Build history of the part. All positions in model axes, mm. A direction names the side the tool comes from. Give positions to 0.01 mm unless a question says otherwise; leave off trailing zeros. Loops run counter-clockwise (first coordinate to the right, second up) from the corner with the lowest first, then second, coordinate; pieces in that order, holes last. Notation, with made-up numbers: (-19, -5.5) - (7, -5.5) arc R24 cw to (7, 26.5) - close; hole circle Ø11 at (50.25, 48). An arc over 180 degrees is marked (long way). Return JSON: item names as keys, results as strings. Group by question number.
1) Slice it at B-B (x = -132.5). List the corners of the cut face in (y, z), and give its area (3 significant figures).
2) Drop flat-ended pins along their axis: pin 1 (0.9 mm diameter, centred on x = -199, z = -195, fed in from +Y); pin 2 (5 mm diameter, centred on x = -5, z = -200, fed in from +Y); pin 3 (9 mm diameter, centred on x = -5, z = -113, fed in from +Y). Give the stop position or say it passes through.
3) Slice it at A-A (z = -147). List the corners of the cut face in (x, y).
4) Mould opens along Z. For faces 6 (the face through (-190, 12, -180)), 7 (the face through (-196, 32, -101)), 8 (the face through (-200, 59, -93)) say: released by +Z, released by -Z, zero draft, split by the parting line, or undercut.
5) Slice it at C-C (y = 41). List the corners of the cut face in (x, z).
6) 3-axis set-ups, long thin cutter, end or side, ignore diameter. For faces 1 (the face through (-188, 15, -90)), 2 (the face through (-191.607, 1.232, -202.733)), 3 (the face through (-186.14, 17.675, -9.86)), 4 (the face through (-101, 0, -100)), 5 (the face through (-201.5, 18.8, -199.8)): which of +Z, -Z, +X, -X, +Y, -Y reach the whole face in a straight line?
7) Drill centre lines: probe 1 along Z at (x, y) = (-5, 1.6); probe 2 along X at (y, z) = (2, -200); probe 3 along Y at (x, z) = (-203.25, -201). Where is each one in solid material? Low to high. Write a range as from..to.
Autodesk Inventor part; units mm, degrees
ref_plane "YZ Plane" through (0, 0, 0) normal (1, 0, 0) x (0, 1, 0)
ref_plane "XZ Plane" through (0, 0, 0) normal (0, 1, 0) x (-1, 0, 0)
ref_plane "XY Plane" through (0, 0, 0) normal (0, 0, 1) x (1, 0, 0)
sketch "スケッチ1" plane through (0, 0, 0) normal (0, 1, 0) x (-1, 0, 0)
  line L0 (0, 0) -> (204, 0)
  line L1 (204, 0) -> (204, -205)
  line L2 (204, -205) -> (0, -205)
  line L3 (0, -205) -> (0, 0)
  dimension "d0" = 204
  dimension "d1" = 205
extrude "押し出し1" add sketch "スケッチ1" along normal blind 5
sketch "スケッチ2" plane through (0, 5, 0) normal (0, 1, 0) x (1, 0, 0)
  line L0 (-204, 205) -> (-204, 0)
  line L1 (0, 205) -> (-204, 205)
  line L2 (-204, 0) -> (-196, 0)
  line L3 (-196, 0) -> (-196, 205)
  line L4 (-196, 205) -> (-204, 205)
  line L5 (-204, 205) -> (-204, 0)
  point P0 (0, 0)
  dimension "d4" = 8
extrude "押し出し2" add sketch "スケッチ2" along normal blind 56
sketch "スケッチ3" plane through (0, 61, 0) normal (0, 1, 0) x (1, 0, 0)
  line L0 (-204, 205) -> (-204, 0)
  line L1 (-196, 0) -> (-196, 205)
  line L2 (-204, 0) -> (-196, 0)
  line L3 (-196, 0) -> (-196, 183)
  line L4 (-196, 183) -> (-204, 183)
  line L5 (-204, 183) -> (-204, 0)
  line L6 (-196, 205) -> (-204, 205)
  point P0 (0, 0)
  point P1 (-200, 183)
  dimension "d7" = 22
extrude "押し出し3" cut sketch "スケッチ3" against normal blind 2 contours L4 L1 L2 L0
sketch "スケッチ4" plane through (0, 61, 0) normal (0, 1, 0) x (1, 0, 0)
  circle A0 centre (-198.5, 195) radius 1.5
  line L0 (-196, 205) -> (-204, 205)
  line L1 (-196, 183) -> (-196, 205)
  line L2 (-204, 205) -> (-204, 183)
  point P0 (0, 0)
  dimension "d10" = 3
  dimension "d11" = 10
  dimension "d13" = 5.5
extrude "押し出し4" cut sketch "スケッチ4" against normal blind 10
sketch "スケッチ5" plane through (-204, 0, -205) normal (-1, 0, 0) x (0, 0, 1)
  circle A0 centre (4, 53) radius 1.5
  circle A1 centre (4, 20) radius 1.5
  line L0 (0, 61) -> (22, 61)
  line L1 (0, 0) -> (0, 61)
  point P0 (205, 0)
  dimension "d16" = 3
  dimension "d17" = 3
  dimension "d18" = 8
  dimension "d19" = 33
  dimension "d24" = 4
extrude "押し出し5" cut sketch "スケッチ5" against normal blind 10
sketch "スケッチ6" plane through (-204, 0, -205) normal (-1, 0, 0) x (0, 0, 1)
  circle A0 centre (4, 53) radius 1.5
  circle A1 centre (4, 53) radius 2.8
  circle A2 centre (4, 20) radius 1.5
  circle A3 centre (4, 20) radius 2.8
  point P0 (205, 0)
  dimension "d22" = 5.6
  dimension "d23" = 5.6
extrude "押し出し6" cut sketch "スケッチ6" against normal blind 2.5
sketch "スケッチ7" plane through (0, 0, 0) normal (0, -1, 0) x (1, 0, 0)
  circle A0 centre (-191, -200) radius 1.5
  circle A1 centre (-101, -200) radius 1.5
  circle A2 centre (-5, -200) radius 1.5
  line L0 (-204, 0) -> (0, 0)
  line L1 (0, 0) -> (0, -205)
  circle A3 centre (-5, -141) radius 1.5
  circle A4 centre (-5, -113) radius 1.5
  line L2 (0, -205) -> (-204, -205)
  dimension "d27" = 3
  dimension "d28" = 3
  dimension "d29" = 3
  dimension "d31" = 5
  dimension "d32" = 96
  dimension "d33" = 90
  dimension "d34" = 3
  dimension "d36" = 3
  dimension "d37" = 5
  dimension "d38" = 59
  dimension "d39" = 28
extrude "押し出し7" cut sketch "スケッチ7" against normal through all
sketch "スケッチ8" plane through (0, 0, 0) normal (0, -1, 0) x (1, 0, 0)
  circle A0 centre (-5, -113) radius 1.5
  circle A1 centre (-5, -113) radius 2.8
  circle A2 centre (-5, -141) radius 1.5
  circle A3 centre (-5, -141) radius 2.8
  circle A4 centre (-5, -200) radius 1.5
  circle A5 centre (-5, -200) radius 2.8
  circle A6 centre (-101, -200) radius 1.5
  circle A7 centre (-101, -200) radius 2.8
  circle A8 centre (-191, -200) radius 1.5
  circle A9 centre (-191, -200) radius 2.8
  point P0 (0, 0)
  dimension "d42" = 5.6
  dimension "d43" = 5.6
  dimension "d44" = 5.6
  dimension "d45" = 5.6
  dimension "d46" = 5.6
extrude "押し出し8" cut sketch "スケッチ8" against normal blind 2.5
sketch "スケッチ9" plane through (0, 5, 0) normal (0, 1, 0) x (1, 0, 0)
  line L0 (0, 205) -> (-204, 205)
  line L1 (0, 0) -> (-5, 0)
  line L2 (-5, 0) -> (-5, 205)
  line L3 (-5, 205) -> (0, 205)
  line L4 (0, 205) -> (0, 0)
  line L5 (-196, 183) -> (-196, 205)
  line L6 (0, 205) -> (-196, 205)
  line L7 (-196, 205) -> (-196, 200)
  line L8 (-196, 200) -> (0, 200)
  line L9 (0, 200) -> (0, 205)
  circle A0 centre (-5, 141) radius 1.5
  circle A1 centre (-5, 141) radius 3.1
  circle A2 centre (-5, 113) radius 1.5
  circle A3 centre (-5, 113) radius 4.1
  circle A4 centre (-5, 200) radius 1.5
  circle A5 centre (-5, 200) radius 3.1
  line L10 (-196, 205) -> (-185.8, 205)
  line L11 (-185.8, 205) -> (-185.8, 196.8)
  line L12 (-185.8, 196.8) -> (-196, 196.8)
  line L13 (-196, 196.8) -> (-196, 205)
  circle A6 centre (-101, 200) radius 1.5
  circle A7 centre (-101, 200) radius 3.1
  point P0 (-5, 137.9)
  point P1 (-5, 117.1)
  point P2 (-5, 108.9)
  point P3 (-185.8, 200)
  point P4 (-8.1, 200)
  point P5 (-5, 196.9)
  point P6 (-5, 144.1)
  point P7 (-104.1, 200)
  point P8 (-97.9, 200)
  point P9 (-99.5, 200)
  point P10 (-102.5, 200)
  dimension "d49" = 5
  dimension "d50" = 5
  dimension "d51" = 6.2
  dimension "d52" = 8.2
  dimension "d53" = 6.2
  dimension "d54" = 10.2
  dimension "d55" = 8.2
  dimension "d58" = 6.2
extrude "押し出し9" cut sketch "スケッチ9" against normal blind 1 contours L4 L8 A5 L2 L0 | L2 A5 L8 A7 L11 L0 | L4 L1 L2 A3 A1 A5 L8 | L11 L8 L5 L0 | A5 L8 A4 L2 | L2 A4 L8 A5 | A5 L2 A4 L8 | L11 L12 L5 L8 | A4 L8 L2 | L2 L8 A4 | L8 A4 L2 A5 | A4 L2 L8 | A7 L8 A6 | L8 A6 A7 | L2 A4 L8 | A3 L2 A2 | L2 A2 A3 | A1 L2 A0 | L2 A0 A1 | A6 L8 | A2 L2 | L2 A2 | A0 L2 | L2 A0 picked at (-100.9397, 200.4964)
sketch "スケッチ10" plane through (0, 5, 0) normal (0, 1, 0) x (1, 0, 0)
  line L0 (-196, 0) -> (-176, 0)
  line L1 (-176, 0) -> (-176, 20)
  line L2 (-176, 20) -> (-196, 20)
  line L3 (-196, 20) -> (-196, 0)
  line L4 (-196, 196.8) -> (-196, 0)
  line L5 (-196, 90) -> (-176, 90)
  line L6 (-176, 90) -> (-176, 100)
  line L7 (-176, 100) -> (-196, 100)
  line L8 (-196, 100) -> (-196, 90)
  line L9 (-196, 170) -> (-176, 170)
  line L10 (-176, 170) -> (-176, 180)
  line L11 (-176, 180) -> (-196, 180)
  line L12 (-196, 180) -> (-196, 170)
  point P0 (0, 0)
  dimension "d59" = 20
  dimension "d60" = 20
  dimension "d61" = 20
  dimension "d62" = 10
  dimension "d63" = 70
  dimension "d64" = 20
  dimension "d65" = 10
  dimension "d66" = 70
extrude "押し出し10" add sketch "スケッチ10" along normal blind 25
sketch "スケッチ11" plane through (-204, 0, 0) normal (0, 0, 1) x (1, 0, 0)
  line L0 (8, 30) -> (8, 5)
  line L1 (28, 5) -> (28, 30)
  line L2 (8, 30) -> (28, 5)
  line L3 (28, 5) -> (28, 30)
  line L4 (28, 30) -> (8, 30)
  point P0 (204, 0)
extrude "押し出し11" cut sketch "スケッチ11" against normal through all
sketch "スケッチ12" plane through (-204, 0, 0) normal (0, 0, 1) x (1, 0, 0)
  circle A0 centre (16, 14) radius 1.5
  line L0 (0, 0) -> (0, 59)
  line L1 (8, 30) -> (8, 5)
  line L2 (8, 5) -> (28, 5)
  point P0 (204, 0)
  dimension "d71" = 3
  dimension "d73" = 8
  dimension "d74" = 9
extrude "押し出し12" cut sketch "スケッチ12" against normal blind 25
fillet "フィレット1" radius 2 2 edges at (-204, 30.5, -205) (0, 2, -205)
fillet "フィレット2" radius 1.5 4 edges at (-203.4142, 0, -204.4142) (-102, 0, -205) (-204, 0, -101.5) (0, 0, -101.5)
fillet "フィレット3" radius 1.5 2 edges at (-196, 5, -135) (-196, 5, -55)
properties part number "オンゲキボタン_bottom_right_3D プリント"
Results:
{
 "1": {"outline": "(0, -203.5) arc R1.5 ccw to (1.5, -205) - (4, -205) - (4, -200) - (5, -200) - (5, 0) - (0, 0) - close", "area": "1,020 mm2"},
 "2": {"pin 1": "y = 51", "pin 2": "y = 4", "pin 3": "y = 5"},
 "3": {"outline": "(-204, 1.5) arc R1.5 ccw to (-202.5, 0) - (-1.5, 0) arc R1.5 ccw to (0, 1.5) - (0, 4) - (-5, 4) - (-5, 5) - (-194.5, 5) arc R1.5 cw to (-196, 6.5) - (-196, 59) - (-204, 59) - close"},
 "4": {"face 6": "released by -Z", "face 7": "undercut", "face 8": "zero draft"},
 "5": {"outline": "(-204, -203) arc R2 ccw to (-202, -205) - (-196, -205) - (-196, 0) - (-204, 0) - close"},
 "6": {"face 1": "+X, +Y", "face 2": "-Y", "face 3": "+Z, -Z, +X, +Y", "face 4": "+Z, -Z, +X, -X, -Y", "face 5": "-X"},
 "7": {"probe 1": "-205..-202.8, -197.2..-143.8, -138.2..-115.8, -110.2..0", "probe 2": "-204..-193.8, -188.2..-103.8, -98.2..-7.8, -2.2..0", "probe 3": "0.2..17.2, 22.8..50.2, 55.8..61"}
}
